Input: part model. Units: mm. Frame: model coordinates. Face numbers are marked on the shaded views. Coordinates: 2 decimals unless noted, no trailing zeros. Write each loop counter-clockwise with the first axis right and the second up, starting at its lowest first coordinate (ties: lowest second). Pieces come first, ordered by that corner, then holes. Notation, with made-up numbers: (54.25, 41) - (63.25, 41) arc R18 cw to (63.25, 74) - close; hole circle Ø9 at (-7.75, 27.5). An arc over 180 degrees is marked (long way). Put each result on its own line as item: value. Start each with the question number.
1. Cut plane C-C, the plane y = -43. Return loops of the section in (x, z).
2. Line query: line 1 (Y direction, x = 230.5, z = 9.25); line 2 (Y direction, x = 46, z = 3.75); line 3 (X direction, y = -38, z = 1.75). Output: solid intervals per line, ascending.
3. Cut plane B-B, the plane z = 6.75. Count the separate pieces of the cut face and the enclosed holes in it, and give its area (3 significant figures).
4. Pull-direction query (Z, two-part tool) for the marked faces 1, 2 and 3; classes: released by +Z, released by -Z, zero draft, split by the parting line, or undercut.
5. Pin query (flat end, axial travel): pin 1 (1 mm diameter, centred on y = -40, z = 3.5, fed in from +X); pin 2 (2.5 mm diameter, centred on x = 238.5, y = -17, fed in from -Z); pin 3 (3 mm diameter, centred on y = -29, z = 3.5, fed in from -X). Return the tip coordinate at first contact, or that it passes through.
6. Cut plane A-A, the plane x = 46. Return loops of the section in (y, z).
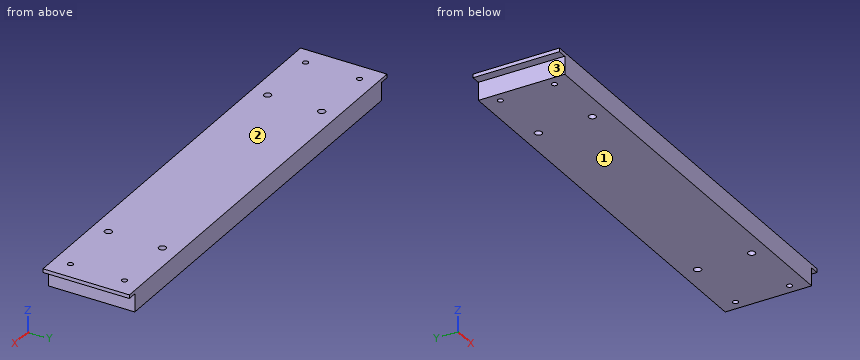
from build123d import *

# Parameters (mm, degrees)
ESQUISSE1_W      = 241
ESQUISSE1_H      = 48
ESQUISSE1_R      = 1.5
ESQUISSE1_R_2    = 2
EXTRUSION1_DEPTH = 12
ESQUISSE2_W      = 5
ESQUISSE2_H      = 10
EXTRUSION2_DEPTH = 49


with BuildPart() as part:
    # Esquisse1 → Extrusion1 (new body)
    with BuildSketch(Plane.XY):
        with Locations((120.5, -24)):
            Rectangle(ESQUISSE1_W, ESQUISSE1_H)
        with Locations((230.5, -39)):
            Circle(ESQUISSE1_R, mode=Mode.SUBTRACT)
        with Locations((10.5, -9)):
            Circle(ESQUISSE1_R, mode=Mode.SUBTRACT)
        with Locations((10.5, -39)):
            Circle(ESQUISSE1_R, mode=Mode.SUBTRACT)
        with Locations((230.5, -9)):
            Circle(ESQUISSE1_R, mode=Mode.SUBTRACT)
        with Locations((195, -39)):
            Circle(ESQUISSE1_R_2, mode=Mode.SUBTRACT)
        with Locations((46, -9)):
            Circle(ESQUISSE1_R_2, mode=Mode.SUBTRACT)
        with Locations((46, -39)):
            Circle(ESQUISSE1_R_2, mode=Mode.SUBTRACT)
        with Locations((195, -9)):
            Circle(ESQUISSE1_R_2, mode=Mode.SUBTRACT)
    extrude(amount=EXTRUSION1_DEPTH)

    # Esquisse2 → Extrusion2 (cut, through all)
    with BuildSketch(Plane(origin=(0, 0, 0), x_dir=(1, 0, 0), z_dir=(0, 1, 0))):
        with Locations((2.5, -5)):
            Rectangle(ESQUISSE2_W, ESQUISSE2_H)
        with Locations((238.5, -5)):
            Rectangle(ESQUISSE2_W, ESQUISSE2_H)
    extrude(amount=-EXTRUSION2_DEPTH, mode=Mode.SUBTRACT)


solid = part.part
Report:
1. outline: (0, 10) - (5, 10) - (5, 0) - (236, 0) - (236, 10) - (241, 10) - (241, 12) - (0, 12) - close
2. line 1: y = -48 to -40.5, -37.5 to -10.5, -7.5 to 0
2. line 2: y = -48 to -41, -37 to -11, -7 to 0
2. line 3: x = 5 to 9.38, 11.62 to 44.27, 47.73 to 193.27, 196.73 to 229.38, 231.62 to 236
3. separate pieces: 1
3. enclosed holes: 8
3. area: 11,000 mm^2
4. face 1: released by -Z
4. face 2: released by +Z
4. face 3: zero draft
5. pin 1: stops at x = 236
5. pin 2: stops at z = 10
5. pin 3: stops at x = 5
6. outline: (-48, 0) - (-41, 0) - (-41, 12) - (-48, 12) - close; (-37, 0) - (-11, 0) - (-11, 12) - (-37, 12) - close; (-7, 0) - (0, 0) - (0, 12) - (-7, 12) - close
